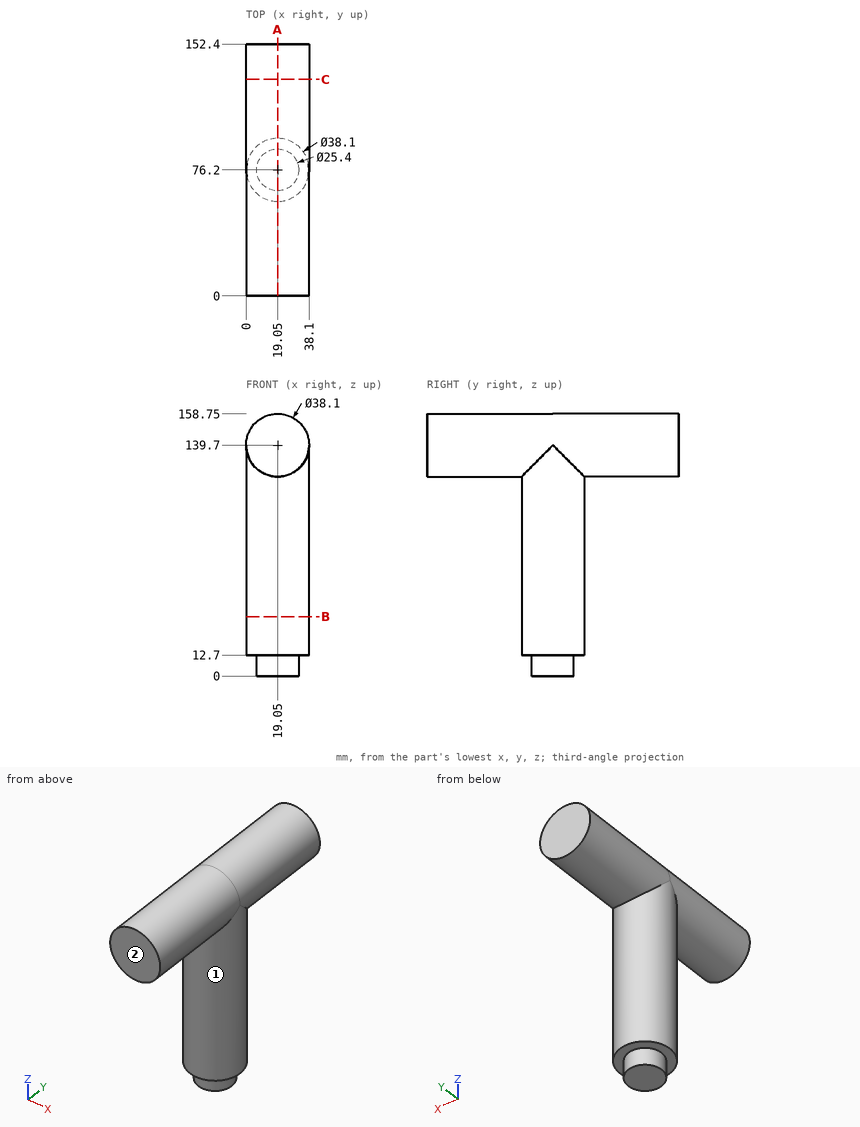
Source: three-view drawing plus pictorial views. Frame: mm from the lowest corner of the part. A direction names the side the tool comes from. Give positions to 0.01 mm unless a question says otherwise; leave off trailing zeros. Write each loop counter-clockwise with the first axis right and the second up, starting at its lowest first coordinate (ties: lowest second). Pieces come first, ordered by that corner, then holes.
(1) Cut plane B-B, the plane z = 36. Return loops of the section in (x, y), then the cut area to 3 significant figures.
(2) Cut plane C-C, the plane y = 131. Return loops of the section in (x, z), then the cut area to 3 significant figures.
(3) Access query for the marked faces 1 and 2. Directions: +Z, -Z, +X, -X, +Y, -Y. A direction counts if a zero-diameter tool reaches every point of the face in a straight line with its end or side. Return the directions, or none.
(4) First-contact query: P1, Ø11.5, axis at x = 23, y = 80.5, coming from the -Z side; P2, Ø2, axis at x = 25.5, z = 94.5, coming from the -Y side; P3, Ø10, axis at x = 22.5, z = 60.5, coming from the -Y side; P4, Ø10, axis at x = 30.5, y = 31.5, coming from the +Z side. Flat tips, straight axial feed; report the tip coordinate or a pass-through.
(5) Ray query, line 1 (Z direction, x = 18, y = 143); line 2 (X direction, y = 79.5, z = 84); line 3 (X direction, y = 52, z = 152.5). Return the intervals inside material, ascending.
(6) Cut plane A-A, the plane x = 19.05. Return loops of the section in (y, z), then the cut area to 3 significant figures.
Values follow:
1. outline: circle Ø38.1 at (19.05, 76.2)
1. area: 1,140 mm2
2. outline: circle Ø38.1 at (19.05, 139.7)
2. area: 1,140 mm2
3. face 1: -Z
3. face 2: +Z, -Z, +X, -X, -Y
4. P1: stops at z = 0
4. P2: stops at y = 57.95
4. P3: stops at y = 57.15
4. P4: stops at z = 157.62
5. line 1: z = 120.68 to 158.72
5. line 2: x = 0.29 to 37.81
5. line 3: x = 4.94 to 33.16
6. outline: (0, 120.65) - (57.15, 120.65) - (57.15, 12.7) - (63.5, 12.7) - (63.5, 0) - (88.9, 0) - (88.9, 12.7) - (95.25, 12.7) - (95.25, 120.65) - (152.4, 120.65) - (152.4, 158.75) - (0, 158.75) - close
6. area: 10,200 mm2
